Source: CAD feature listing. Evaluate the final solid. Frame: model axes, mm. Face numbers are marked on the shaded views. Coordinates: 2 decimals unless noted, no trailing zeros. Loops run counter-clockwise (first coordinate to the right, second up) from the corner with the lowest first, then second, coordinate; pieces in that order, holes last. Notation, with made-up numbers: (87.5, -30) -> (108.5, -30) arc R10 cw to (108.5, -23) -> close; hole circle Ø9 at (-20, -22). An arc over 180 degrees is marked (long way). Answer as a JSON object with one key per item and string values. Group by question number.
from build123d import *

# Parameters (mm, degrees)
SKETCH1_R           = 5
BOSS_EXTRUDE1_DEPTH = 4


with BuildPart() as part:
    # Sketch1 → Boss-Extrude1 (new body)
    with BuildSketch(Plane(origin=(0, 0, 0), x_dir=(0, 0, -1), z_dir=(1, 0, 0))):
        with BuildLine():
            Line((-31.850752253, 36.420784179), (-7.861259629, -5.130235893))
            ThreePointArc((-7.861259629, -5.130235893), (-7.861259629, -16.324481088), (-17.555760345, -21.921603686))
            Line((-17.555760345, -21.921603686), (-65.534745592, -21.921603686))
            ThreePointArc((-65.534745592, -21.921603686), (-75.229246307, -16.324481088), (-75.229246307, -5.130235893))
            Line((-75.229246307, -5.130235893), (-51.239753683, 36.420784179))
            ThreePointArc((-51.239753683, 36.420784179), (-41.545252968, 42.017906776), (-31.850752253, 36.420784179))
        make_face()
        with Locations((-41.545252968, 30.823661581)):
            Circle(SKETCH1_R, mode=Mode.SUBTRACT)
        with Locations((-17.555760345, -10.727358491)):
            Circle(SKETCH1_R, mode=Mode.SUBTRACT)
        with Locations((-65.534745592, -10.727358491)):
            Circle(SKETCH1_R, mode=Mode.SUBTRACT)
    extrude(amount=BOSS_EXTRUDE1_DEPTH)


solid = part.part
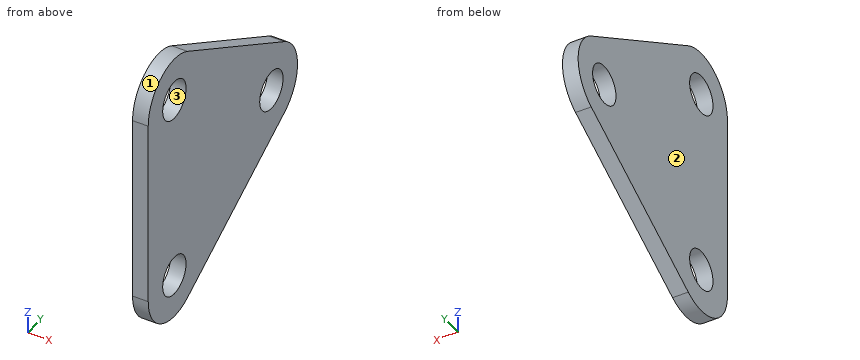
1. Section query B-B on y = 28.5. Return loops of the section in (x, z).
2. Section query D-D on y = 15.5. Return loops of the section in (x, z), then the cut area to 3 significant figures.
3. Ray query, L1, parallel to Z at x = 1.1, y = -11.5; L2, parallel to Z at x = 1, y = -8.5; L3, parallel to Y at x = 3.15, z = 20. Return the intervals inside material, ascending.
4. Section query A-A on z = 21. Return loops of the section in (x, y).
5. Section query C-C on x = 2.45. Return loops of the section in (y, z), then the cut area to 3 significant figures.
6. Mould query, pull axis Z, two halves, no side actions, for the marked faces 1, 2 and 3. Classes: pulls with the +Z half, pulls with the -Z half, needs draft (parallel to the pull), parting line crosses it, or undercut.
7. Pin query (flat end, axial travel): pin 1 Ø1.5 at (x, z) = (2, 29.5) entering from +Y; pin 2 Ø13 at (y, z) = (-10.73, 65.53) entering from +X; pin 3 Ø1 at (x, z) = (3.5, 67) entering from -Y. Return the tip coordinate at first contact, or that it passes through.
Solved:
{
 "1": {"outline": "(0, 27.28) -> (4, 27.28) -> (4, 37.12) -> (0, 37.12) -> close; (0, 45.97) -> (4, 45.97) -> (4, 55.81) -> (0, 55.81) -> close"},
 "2": {"outline": "(0, 19.77) -> (4, 19.77) -> (4, 63.32) -> (0, 63.32) -> close", "area": "174 mm^2"},
 "3": {"L1": "6.39 to 12.62, 22.5 to 60.59, 70.47 to 76.7", "L2": "6.59 to 13.08, 22.03 to 61.06, 70.01 to 76.51", "L3": "-21.92 to -15.09, -6.37 to 15.89"},
 "4": {"outline": "(0, -21.92) -> (4, -21.92) -> (4, -14.35) -> (0, -14.35) -> close; (0, -7.1) -> (4, -7.1) -> (4, 17.63) -> (0, 17.63) -> close"},
 "5": {"outline": "(-21.92, 17.56) arc R11.19 ccw to (-5.13, 7.86) -> (36.42, 31.85) arc R11.19 ccw to (36.42, 51.24) -> (-5.13, 75.23) arc R11.19 ccw to (-21.92, 65.53) -> close; hole circle Ø10 at (-10.73, 17.56); hole circle Ø10 at (-10.73, 65.53); hole circle Ø10 at (30.82, 41.55)", "area": "2,770 mm^2"},
 "6": {"face 1": "pulls with the +Z half", "face 2": "needs draft", "face 3": "undercut"},
 "7": {"pin 1": "y = 33.65", "pin 2": "x = 4", "pin 3": "y = -21.88"}
}
